Autodesk Inventor part; units mm, degrees
ref_plane "YZ Plane" through (0, 0, 0) normal (1, 0, 0) x (0, 1, 0)
ref_plane "XZ Plane" through (0, 0, 0) normal (0, 1, 0) x (-1, 0, 0)
ref_plane "XY Plane" through (0, 0, 0) normal (0, 0, 1) x (1, 0, 0)
sketch "Эскиз1" plane through (0, 0, 0) normal (0, 0, 1) x (1, 0, 0)
  line L0 (-34.95, 71) -> (-39.5, 71)
  line L1 (-39.5, 71) -> (52.5, 71)
  line L2 (52.5, 71) -> (52.5, 51)
  line L3 (-19.5, -21) -> (-39.5, -21)
  line L4 (-39.5, -21) -> (-39.5, 71)
  line L5 (-21, 66.8757) -> (-21, 32.8243) construction
  line L6 (-19.5, 71) -> (22.5, 71)
  line L7 (22.5, 51) -> (22.5, 29)
  line L8 (22.5, 29) -> (-19.5, 29)
  line L9 (-19.5, 29) -> (-19.5, 71)
  line L10 (-19.5, 29) -> (22.5, 29)
  line L11 (-19.5, -21) -> (-19.5, 29)
  line L12 (22.5, 29) -> (22.5, 51)
  line L13 (22.5, 51) -> (52.5, 51)
  dimension "d14" = 92
  dimension "d20" = 20
  dimension "d21" = 42
  dimension "d22" = 42
  dimension "d24" = 92
  dimension "d25" = 30
extrude "Выдавливание1" add sketch "Эскиз1" along normal blind 4
sketch "Эскиз2" plane through (0, 0, 4) normal (0, 0, 1) x (1, 0, 0)
  circle A0 centre (0.15, 49.85) radius 11
  line L0 (52.5, 51) -> (52.5, 71)
  line L1 (52.5, 61) -> (-39.5, 61) construction
  line L2 (-39.5, 71) -> (-39.5, -21)
  line L3 (-39.5, -21) -> (-19.5, -21)
  line L4 (-29.5, -21) -> (-29.5, 71) construction
  line L5 (52.5, 71) -> (-39.5, 71)
  circle A1 centre (44.5, 61) radius 2.1
  circle A2 centre (28.5, 61) radius 2.1
  circle A3 centre (-15.35, 34.35) radius 1.25
  circle A4 centre (15.65, 34.35) radius 1.25
  circle A5 centre (15.65, 65.35) radius 1.25
  circle A6 centre (-15.35, 65.35) radius 1.25
  line L6 (-39.5, 71) -> (-29.5, 61) construction
  circle A7 centre (-29.5, -13) radius 2.1
  circle A8 centre (-29.5, 3) radius 2.1
  dimension "d26" = 4.2
  dimension "d27" = 4.2
  dimension "d28" = 8
  dimension "d29" = 16
extrude "Выдавливание2" cut sketch "Эскиз2" against normal blind 4
fillet "Сопряжение1" radius 4 8 edges at (-39.5, -21, 2) (-19.5, -21, 2) (-19.5, 29, 2) (22.5, 29, 2) (22.5, 51, 2) (52.5, 51, 2) (52.5, 71, 2) (-39.5, 71, 2)
properties part number "креп_мотора"
Input: part model. Units: mm. Frame: model coordinates. A direction names the side the tool comes from. Round coordinates to 2 decimals unless told otherwise and drop trailing zeros. Loops run counter-clockwise (first coordinate to the right, second up) from the corner with the lowest first, then second, coordinate; pieces in that order, holes last. Notation, with made-up numbers: (86.25, 19.25) -> (102.25, 19.25) arc R26 cw to (102.25, 56.25) -> close; hole circle Ø7 at (53.5, -13.5). An arc over 180 degrees is marked (long way). Write each question's results on one line, items separated by ' | '.
1. Mould query, pull axis Y, two halves, no side actions, for faces 1 (the face through (-20.703, -19.859, 2.028)), 2 (the face through (51.359, 69.797, 2.028)), 3 (the face through (-31.6, -12.91, 2.03)). Classes: +Y half, -Y half, draft (parallel to the pull), parting line (faces both ways), or undercut.
Geometry results:
face 1: -Y half | face 2: +Y half | face 3: undercut
2. First-contact query: P1, Ø2, axis at x = 16, z = 1.5, coming from the -Y side; P2, Ø2, axis at y = 43, z = 1, coming from the +X side; P3, Ø2, axis at y = 13, z = 1.5, coming from the +X side. Flat tips, straight axial feed; report the tip coordinate or a pass-through.
Geometry results:
P1: y = 29 | P2: x = 22.5 | P3: x = -19.5
3. Section A-A (x = 28.5). Return loops of the section in (y, z).
Geometry results:
outline: (51, 0) -> (58.9, 0) -> (58.9, 4) -> (51, 4) -> close; (63.1, 0) -> (71, 0) -> (71, 4) -> (63.1, 4) -> close
4. Set-up query: faces 4 (the face through (2, 29, 2)), 5 (the face through (6.1, 59.1, 2)). Return all of +Z, -Z, +X, -X, +Y, -Y with unobstructed straight access to the full face (end or side cutting, diameter ignored); none if empty.
Geometry results:
face 4: +Z, -Z, +X, -Y | face 5: +Z, -Z
5. Ray query, line 1 (Y direction, x = -15.35, z = 2.9); line 2 (X direction, y = 65.35, z = 2.4); line 3 (Y direction, x = -29.5, z = 1.35). Return the intervals inside material, ascending. Write a range as from..to.
Geometry results:
line 1: 29..33.1, 35.6..64.1, 66.6..71 | line 2: -39.5..-16.6, -14.1..14.4, 16.9..52.5 | line 3: -21..-15.1, -10.9..0.9, 5.1..71
6. Section D-D (y = 44). Return loops of the section in (x, z).
Geometry results:
outline: (-39.5, 0) -> (-9.17, 0) -> (-9.17, 4) -> (-39.5, 4) -> close; (9.47, 0) -> (22.5, 0) -> (22.5, 4) -> (9.47, 4) -> close
7. Section B-B (z = 3). State how many separate pieces and enclosed holes the cut face has, and give its area (3 significant figures).
Geometry results:
separate pieces: 1 | enclosed holes: 9 | area: 3,740 mm2
8. Section C-C (y = 34.35). Return loops of the section in (x, z).
Geometry results:
outline: (-39.5, 0) -> (-16.6, 0) -> (-16.6, 4) -> (-39.5, 4) -> close; (-14.1, 0) -> (14.4, 0) -> (14.4, 4) -> (-14.1, 4) -> close; (16.9, 0) -> (22.5, 0) -> (22.5, 4) -> (16.9, 4) -> close
